Design review of the part built by this model. Coordinates are the model's own, in mm. A direction names the side the tool comes from. Round coordinates to 2 decimals unless told otherwise and drop trailing zeros. Order: outer loops, then holes, each group sorted by start corner. A loop starts at its lowest first (then second) coordinate and runs counter-clockwise, first axis right, second up. Notation, with made-up numbers: (84.25, 37) - (112.25, 37) arc R21 cw to (112.25, 67) - close; hole circle Ø3 at (44.25, 59). An arc over 180 degrees is marked (long way). Write item = value, one per line.
Autodesk Inventor part; units mm, degrees
ref_plane "YZ Plane" through (0, 0, 0) normal (1, 0, 0) x (0, 1, 0)
ref_plane "XZ Plane" through (0, 0, 0) normal (0, 1, 0) x (-1, 0, 0)
ref_plane "XY Plane" through (0, 0, 0) normal (0, 0, 1) x (1, 0, 0)
sketch "Sketch1" plane through (0, 0, 0) normal (0, 1, 0) x (-1, 0, 0)
  line L0 (0, 0) -> (-12, 0)
  line L1 (-12, 0) -> (-12, -17)
  line L2 (-12, -17) -> (0, -17)
  line L3 (0, -17) -> (0, 0)
  line L4 (0, 0) -> (2, 0)
  line L5 (2, 0) -> (2, 2)
  line L6 (2, 2) -> (-12, 2)
  line L7 (-12, 2) -> (-12, -19)
  line L8 (-12, -19) -> (2, -19)
  line L9 (2, -19) -> (2, 2)
  dimension "d0" = 12
  dimension "d1" = 17
  dimension "d2" = 2
  dimension "d3" = 2
  dimension "d4" = 21
extrude "Extrusion1" add sketch "Sketch1" along normal blind 4
sketch "Sketch3" plane through (0, 4, 0) normal (0, 1, 0) x (1, 0, 0)
  line L0 (12, -2) -> (12, 19)
  line L1 (0, 0) -> (12, 0)
  line L2 (12, 0) -> (12, 17)
  line L3 (12, 17) -> (0, 17)
  line L4 (0, 17) -> (0, 0)
  dimension "d7" = 17
extrude "Extrusion2" cut sketch "Sketch3" against normal blind 2.5
sketch "Sketch4" plane through (0, 4, 0) normal (1, 0, 0) x (0, 0, -1)
  line L0 (-2, 0) -> (0, 0)
  line L1 (17, 0) -> (17, -2.5)
  line L2 (0, 0) -> (17, 0)
  line L3 (17, 0) -> (17, -1.5)
  line L4 (17, -1.5) -> (0, -1.5)
  line L5 (0, -1.5) -> (0, 0)
  point P0 (0, -4)
  dimension "d10" = 1.5
extrude "Extrusion3" add sketch "Sketch4" along normal blind 0.5
sketch "Sketch5" plane through (0, 1.5, -17) normal (0, 0, 1) x (1, 0, 0)
  line L0 (12, 2.5) -> (12, 0)
  line L1 (0.5, 2.5) -> (12, 2.5)
  line L2 (12, 2.5) -> (12, 1)
  line L3 (12, 1) -> (0.5, 1)
  line L4 (0.5, 1) -> (0.5, 2.5)
  point P0 (0, -1.5)
  dimension "d13" = 1.5
extrude "Extrusion4" add sketch "Sketch5" along normal blind 0.5
sketch "Sketch6" plane through (12, 1.5, 0) normal (0, 0, -1) x (-1, 0, 0)
  line L0 (14, 2.5) -> (0, 2.5)
  line L1 (12, 1) -> (11.5, 1)
  line L2 (0, 2.5) -> (11.5, 2.5)
  line L3 (11.5, 2.5) -> (11.5, 1)
  line L4 (11.5, 1) -> (0, 1)
  line L5 (0, 1) -> (0, 2.5)
  point P0 (12, -1.5)
  dimension "d20" = 1.5
extrude "Extrusion5" add sketch "Sketch6" along normal blind 0.5
sketch "Sketch7" plane through (12, 0, 2) normal (1, 0, 0) x (0, 0, -1)
  line L0 (19, 2.5) -> (19, 1.5)
  line L1 (19, 1.5) -> (2, 1.5)
  line L2 (2, 1.5) -> (2, 0)
  line L3 (2, 0) -> (19, 0)
  line L4 (19, 0) -> (19, 1.5)
extrude "Extrusion6" cut sketch "Sketch7" against normal blind 3.5
sketch "Sketch8" plane through (-2, 0, -19) normal (-1, 0, 0) x (0, 0, 1)
  line L0 (0, 0) -> (21, 0)
  line L1 (21, 0) -> (21, 4)
  line L2 (0, 4) -> (21, 4)
  line L3 (0, 0) -> (0, 4)
  point P0 (19, 0)
extrude "Extrusion7" add sketch "Sketch8" along normal blind 4.5
chamfer "Chamfer2" distance 6.5 angle 45 1 edges at (-6.5, 2, 2)
sketch "Sketch16" plane through (0, 2.5, -17) normal (0, 0, 1) x (1, 0, 0)
  line L0 (12, 0) -> (0, 0)
  line L1 (0, 0) -> (0, -1)
  line L2 (0, -1) -> (8.5, -1)
  line L3 (8.5, -1) -> (8.5, -2.5)
  line L4 (12, -2.5) -> (8.5, -2.5)
  line L5 (12, 0) -> (12, -2.5)
  point P0 (0, -2.5)
extrude "Extrusion14" cut sketch "Sketch16" against normal blind 0.5
sketch "Sketch17" plane through (12, 2.5, 0) normal (0, 0, -1) x (-1, 0, 0)
  line L0 (12, 0) -> (0, 0)
  line L1 (0, -2.5) -> (0, 0)
  line L2 (3.5, -2.5) -> (0, -2.5)
  line L3 (3.5, -2.5) -> (3.5, -1)
  line L4 (3.5, -1) -> (12, -1)
  line L5 (12, 0) -> (12, -1)
  point P0 (12, -2.5)
extrude "Extrusion15" cut sketch "Sketch17" against normal blind 0.5
sketch "Sketch18" plane through (0.5, 2.5, -16.5) normal (0, -1, 0) x (1, 0, 0)
  line L0 (-0.5, -1) -> (-0.5, 17)
  line L1 (-0.5, -1) -> (11.5, -1)
  line L2 (11.5, 0) -> (11.5, -1)
  line L3 (0, 0) -> (11.5, 0)
  line L4 (0, 16) -> (0, 0)
  line L5 (11.5, 16) -> (0, 16)
  line L6 (11.5, 17) -> (11.5, 16)
  line L7 (11.5, 17) -> (-0.5, 17)
  point P0 (-0.5, 16.5)
extrude "Extrusion16" cut sketch "Sketch18" against normal blind 0.5
chamfer "Chamfer3" distance 6.5 angle 45 1 edges at (-6.5, 2, -19)
sketch "Sketch19" plane through (0, 0, 0) normal (0, -1, 0) x (1, 0, 0)
  line L0 (0, -19) -> (-6.5, -12.5)
  line L1 (12, -19) -> (0, -19)
  line L2 (12, -17.5) -> (12, -19)
  line L3 (12, -17.5) -> (8.5, -17.5)
  line L4 (8.5, -17.5) -> (8.5, 0.5)
  line L5 (8.5, 0.5) -> (12, 0.5)
  line L6 (12, 2) -> (12, 0.5)
  line L7 (12, 2) -> (0, 2)
  line L8 (-6.5, -4.5) -> (0, 2)
  line L9 (-6.5, -12.5) -> (-6.5, -4.5)
  point P0 (0, 0)
extrude "Extrusion17" add sketch "Sketch19" along normal blind 2
sketch "Sketch22" plane through (0, 1.5, -16.5) normal (0, 0, 1) x (1, 0, 0)
  line L0 (0.5, 1.5) -> (12, 1.5)
  line L1 (12, 1.5) -> (12, 2.5)
  line L2 (12, 2.5) -> (0.5, 2.5)
  line L3 (0.5, 1.5) -> (0.5, 2.5)
  point P0 (0, -1.5)
extrude "Extrusion20" cut sketch "Sketch22" against normal blind 0.5
sketch "Sketch23" plane through (12, 1.5, -0.5) normal (0, 0, -1) x (-1, 0, 0)
  line L0 (0, 1.5) -> (11.5, 1.5)
  line L1 (11.5, 2.5) -> (11.5, 1.5)
  line L2 (11.5, 2.5) -> (0, 2.5)
  line L3 (0, 2.5) -> (0, 1.5)
  point P0 (12, -1.5)
extrude "Extrusion21" cut sketch "Sketch23" against normal blind 0.5
sketch "Sketch24" plane through (-6.5, 0, -19) normal (-1, 0, 0) x (0, 0, 1)
  circle A0 centre (10.5, 1) radius 2.6
  point P0 (19, 0)
  dimension "d79" = 5.2
extrude "Extrusion22" cut sketch "Sketch24" against normal blind 5
sketch "Sketch25" plane through (-1.5, 1, -8.5) normal (-1, 0, 0) x (0, 0, 1)
  circle A0 centre (0, 0) radius 2.6
  line L0 (0, 0) -> (0, -1.5)
  line L1 (0, -1.5) -> (2.1237, -1.5)
  line L2 (0, -1.5) -> (-2.1237, -1.5)
  arc A1 (-2.1237, -1.5) -> (2.1237, -1.5) centre (0, 0) ccw
  arc A2 (2.0494, 1.6) -> (-2.0494, 1.6) centre (0, 0) ccw
  line L3 (0, 0) -> (0, 1.5)
  line L4 (2.1237, 1.5) -> (-2.1237, 1.5)
  line L5 (-2.6, 0) -> (2.6, 0)
  point P0 (8.5, -1)
  dimension "d88" = 1.5
  dimension "d89" = 1.5
  dimension "d90" = 5.2
extrude "Extrusion23" add sketch "Sketch25" along normal blind 5 contours L4 A0 | A0 L2 L1
sketch "Sketch26" plane through (0, 1.5, 0) normal (0, 1, 0) x (1, 0, 0)
  circle A0 centre (2.5, 2) radius 1.1
  line L0 (0, -0.5) -> (0, 17.5)
  line L1 (0, -0.5) -> (8.5, -0.5)
  line L2 (8.5, -0.5) -> (8.5, 17.5)
  line L3 (8.5, 8.5) -> (0, 8.5)
  circle A1 centre (2.5, 15) radius 1.1
  point P0 (0, 0)
  dimension "d91" = 2.2
  dimension "d92" = 2.5
  dimension "d93" = 2.5
extrude "Extrusion24" cut sketch "Sketch26" against normal blind 3.5 contours A0 | A1
sketch "Sketch27" plane through (8.5, 0, 2) normal (1, 0, 0) x (0, 0, -1)
  line L0 (19.5, -2) -> (19.5, 1.5)
  line L1 (1.5, 1.5) -> (19.5, 1.5)
  line L2 (1.5, 1.5) -> (1.5, -2)
  line L3 (19.5, -2) -> (1.5, -2)
  point P0 (2, 0)
extrude "Extrusion25" cut sketch "Sketch27" against normal blind 1
properties part number "sensorHolder"
1) We need section C-C on z = -15. Write out the cut boundary in (x, y).
Findings:
outline = (-4, -2) - (1.4, -2) - (1.4, 1.5) - (0, 1.5) - (0, 3) - (0.5, 3) - (0.5, 4) - (-4, 4) - close; (3.6, -2) - (7.5, -2) - (7.5, 1.5) - (3.6, 1.5) - close
2) Clearance check with flat-ended pins moving along their axes: pin 1 Ø1 at (x, z) = (2, -11) entering from +Y; pin 2 Ø0.8 at (y, z) = (2.5, -6.5) entering from +X; pin 3 Ø2.5 at (y, z) = (1, -9) entering from -X. State where each tip first meets the part, or that it passes through.
Findings:
pin_1 = 1.5
pin_2 = 0
pin_3 = -1.5
3) For faces 1 (the flat face through (6, 1, -19)), 2 (the flat face through (-4, -0.5, -8)), 3 (the flat face through (6.3, 3.5, 0)), 4 (the flat face through (7, 2, -17.5)), 5 (the cylindrical face through (3.516, -0.226, -1.579)), list the 3-axis set-ups (+Z, -Z, +X, -X, +Y, -Y) from which the entire face can be reached by the end or side of a thin tool; tool diameter is ignored.
Findings:
face_1 = -Z, +X, -X, +Y, -Y
face_2 = -X
face_3 = +X, +Y
face_4 = +X
face_5 = +Y, -Y
4) We need section D-D on z = -4. Write out the cut boundary in (x, y).
Findings:
outline = (-6, -2) - (7.5, -2) - (7.5, 1.5) - (0, 1.5) - (0, 3) - (0.5, 3) - (0.5, 4) - (-6, 4) - close
5) To check wall thickness, follow L1, parallel to Z at x = 2.5, y = -0.15; L2, parallel to Z at x = 8, y = 0.7; L3, parallel to Z at x = 1.75, y = -0.8. State the ranges of each line that lie inside material, in increasing order. Write a range as from..to.
Findings:
L1 = -19..-16.1, -13.9..-3.1, -0.9..2
L2 = -19..-17.5, 0.5..2
L3 = -19..-15.8, -14.2..-2.8, -1.2..2
6) We need section B-B on x = 10.25. Write out the cut boundary in (y, z), and give its area (3 significant figures).
Findings:
outline = (-2, -19) - (4, -19) - (4, -17) - (3, -17) - (3, -17.5) - (-2, -17.5) - close; (-2, 0.5) - (3, 0.5) - (3, 0) - (4, 0) - (4, 2) - (-2, 2) - close
area = 19.0 mm^2
7) The part is to be moulded in two halves that separate along Y. For faces 6 (the flat face through (12, 1, -18)), 7 (the flat face through (3, -2, -8)), 8 (the flat face through (7, 2, 0.5)), say which applies: released by +Y, released by -Y, zero draft, split by the parting line, or undercut.
Findings:
face_6 = zero draft
face_7 = released by -Y
face_8 = undercut
8) We need section A-A on x = 2.5. Write out the cut boundary in (y, z).
Findings:
outline = (-2, -19) - (4, -19) - (4, -17) - (3, -17) - (3, -17.5) - (1.5, -17.5) - (1.5, -16.1) - (-2, -16.1) - close; (-2, -13.9) - (1.5, -13.9) - (1.5, -3.1) - (-2, -3.1) - close; (-2, -0.9) - (1.5, -0.9) - (1.5, 0.5) - (3, 0.5) - (3, 0) - (4, 0) - (4, 2) - (-2, 2) - close
